Model file for the job. Use its own axes, mm. Face numbers are marked on the shaded views. Coordinates: 2 decimals unless noted, no trailing zeros. Write each loop counter-clockwise with the first axis right and the second up, starting at its lowest first coordinate (ties: lowest second). Pieces come first, ordered by that corner, then holes. Notation, with made-up numbers: M 39.25,65.5 L 66.25,65.5 A16 cw 66.25,83.5 Z; hole C -5.75,48 d10. An arc over 180 degrees is marked long. Put each result on its own line as item: value. Start each with the question number.
Q1. Pull direction X, two halves, no side cores. Call the marked faces 1 and 2: pulls with the +X half, pulls with the -X half, needs draft (parallel to the pull), parting line crosses it, or undercut.
Q2. Cut at B-B (z = -2). Write the cut outline in (x, y) (1 decimal), then the cut area to 3 significant figures.
Q3. Drill centre lines: line 1 along X through (y, z) = (24, 1.95); line 2 along Y through (x, z) = (-7, 0.35); line 3 along X through (y, z) = (3, 0.7). Where is each one in solid material? Low to high.
Q4. Cut at C-C (y = -7). Write the cut outline in (x, z).
Q5. Cut at A-A (x = 27). Write the cut outline in (y, z), then the cut area to 3 significant figures.
Q6. Drop flat-ended pins along their axis: pin 1 (1.9 mm diameter, centred on x = -35.56, y = -24.19, fed in from -Z); pin 2 (8 mm diameter, centred on x = -24.5, y = -19, fed in from -Z). Give the stop position or say it passes through.
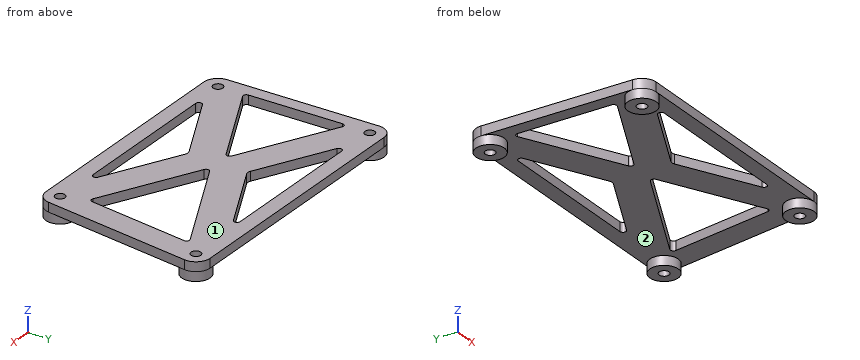
Autodesk Inventor part; units mm, degrees
ref_plane "YZ Plane" through (0, 0, 0) normal (1, 0, 0) x (0, 1, 0)
ref_plane "XZ Plane" through (0, 0, 0) normal (0, 1, 0) x (-1, 0, 0)
ref_plane "XY Plane" through (0, 0, 0) normal (0, 0, 1) x (1, 0, 0)
sketch "Sketch1" plane through (0, 0, 0) normal (0, 0, 1) x (1, 0, 0)
  circle A0 centre (-36.83, 24.0665) radius 1.5875
  circle A1 centre (45.72, 24.0665) radius 1.5875
  circle A2 centre (39.37, -24.1935) radius 1.5875
  circle A3 centre (-35.56, -24.1935) radius 1.5875
  arc A4 (-36.83, 28.654) -> (-41.4159, 23.9458) centre (-36.83, 24.0665) ccw
  arc A5 (-40.1459, -24.3142) -> (-35.56, -28.781) centre (-35.56, -24.1935) ccw
  arc A6 (39.37, -28.781) -> (43.9183, -24.792) centre (39.37, -24.1935) ccw
  arc A7 (50.2683, 23.468) -> (45.72, 28.654) centre (45.72, 24.0665) ccw
  line L0 (50.2683, 23.468) -> (43.9183, -24.792)
  line L1 (39.37, -28.781) -> (-35.56, -28.781)
  line L2 (-40.1459, -24.3142) -> (-41.4159, 23.9458)
  line L3 (-36.83, 28.654) -> (45.72, 28.654)
  point P0 (0, 0)
  dimension "d0" = 3
  dimension "d1" = 3
  dimension "d2" = 3
  dimension "d3" = 3
extrude "Main body" add sketch "Sketch1" along normal blind 3
sketch "Sketch3" plane through (0, 0, 0) normal (0, 0, -1) x (-1, 0, 0)
  circle A0 centre (35.56, -24.1935) radius 1.5875
  circle A1 centre (-39.37, -24.1935) radius 1.5875
  circle A2 centre (-45.72, 24.0665) radius 1.5875
  circle A3 centre (36.83, 24.0665) radius 1.5875
  circle A4 centre (35.56, -24.1935) radius 4.5875
  circle A5 centre (-39.37, -24.1935) radius 4.5875
  circle A6 centre (-45.72, 24.0665) radius 4.5875
  circle A7 centre (36.83, 24.0665) radius 4.5875
  point P0 (0, 0)
  dimension "d7" = 3
  dimension "d8" = 3
  dimension "d9" = 3
  dimension "d10" = 3
extrude "Standoff" add sketch "Sketch3" along normal blind 3
sketch "Sketch4" plane through (0, 0, 0) normal (0, 0, -1) x (-1, 0, 0)
  line L0 (28.3461, 23.654) -> (-28.3461, 23.654)
  line L1 (-28.3461, 23.654) -> (0, 9.4725)
  line L2 (0, 9.4725) -> (28.3461, 23.654)
  line L3 (37.0154, 16.8096) -> (3.4163, 0)
  line L4 (3.4163, 0) -> (36.1422, -16.3727)
  line L5 (36.1422, -16.3727) -> (37.0154, 16.8096)
  line L6 (28.5999, -23.781) -> (0, -9.4725)
  line L7 (0, -9.4725) -> (-28.5999, -23.781)
  line L8 (-28.5999, -23.781) -> (28.5999, -23.781)
  line L9 (35.56, -28.781) -> (-39.37, -28.781)
  line L10 (-45.72, 28.654) -> (36.83, 28.654)
  line L11 (-3.4163, 0) -> (-41.6219, 19.1142)
  line L12 (-41.6219, 19.1142) -> (-36.9025, -16.7531)
  line L13 (-36.9025, -16.7531) -> (-3.4163, 0)
  line L14 (-3.4163, 0) -> (3.4163, 0) construction
  line L15 (0, -9.4725) -> (0, 9.4725) construction
  line L16 (41.4159, 23.9458) -> (40.1459, -24.3142) construction
  line L17 (-43.9183, -24.792) -> (-50.2683, 23.468) construction
  point P0 (0, 0)
  dimension "d13" = 5
  dimension "d14" = 5
  dimension "d15" = 10
  dimension "d16" = 10
  dimension "d17" = 10
  dimension "d18" = 10
extrude "Extrusion3" cut sketch "Sketch4" against normal up to surface (3 mm away)
fillet "Fillet1" radius 1 8 edges at (-28.3461, 23.654, 1.5) (28.3461, 23.654, 1.5) (41.6219, 19.1142, 1.5) (36.9025, -16.7531, 1.5) (-28.5999, -23.781, 1.5) (-36.1422, -16.3727, 1.5) (-37.0154, 16.8096, 1.5) (28.5999, -23.781, 1.5)
fillet "Fillet2" radius 2 2 edges at (0, -9.4725, 1.5) (0, 9.4725, 1.5)
fillet "Fillet3" radius 1 2 edges at (-3.4163, 0, 1.5) (3.4163, 0, 1.5)
equation "\"d1\" = d0"
equation "\"d2\" = d0"
equation "\"d3\" = d0"
equation "\"d8\" = d7"
equation "\"d9\" = d7"
equation "\"d10\" = d7"
equation "\"d14\" = d13"
equation "\"d16\" = d15"
equation "\"d17\" = d15"
equation "\"d18\" = d15"
properties part number "RampsMount"
Computed values:
1. face 1: needs draft
1. face 2: undercut
2. outline: C -36.8,24.1 d9.2; C -35.6,-24.2 d9.2; C 39.4,-24.2 d9.2; C 45.7,24.1 d9.2; hole C -36.8,24.1 d3.2; hole C -35.6,-24.2 d3.2; hole C 39.4,-24.2 d3.2; hole C 45.7,24.1 d3.2
2. area: 233 mm2
3. line 1: -41.42 to -38.42, -35.24 to 44.13, 47.31 to 50.31
3. line 2: -28.78 to -23.78, -12.97 to -1.79, 1.79 to 12.97, 23.65 to 28.65
3. line 3: -40.86 to -36.65, -9.41 to 9.41, 39.5 to 47.58
4. outline: M -40.6,0 L -36.39,0 L -36.39,3 L -40.6,3 Z; M -17.41,0 L 17.41,0 L 17.41,3 L -17.41,3 Z; M 38.19,0 L 46.26,0 L 46.26,3 L 38.19,3 Z
5. outline: M -28.78,0 L -11.8,0 L -11.8,3 L -28.78,3 Z; M 11.8,0 L 28.65,0 L 28.65,3 L 11.8,3 Z
5. area: 102 mm2
6. pin 1: through
6. pin 2: z = 0
